Geometry: see drawing. Coordinates: mm, zero at the bounding-box minimum. A direction names the side the tool comes from. Give positions to 0.01 mm unless a question says otherwise; leave off trailing zeros. Loops run counter-clockwise (first coordinate to the right, second up) from the corner with the lowest first, then second, coordinate; pieces in that order, holes last. Notation, with made-up numbers: M -36,67 L -7,67 A24 ccw -7,90 Z; hole C -38,47.25 d6. An arc over 180 degrees is marked long. Put each result on its own line as item: value.
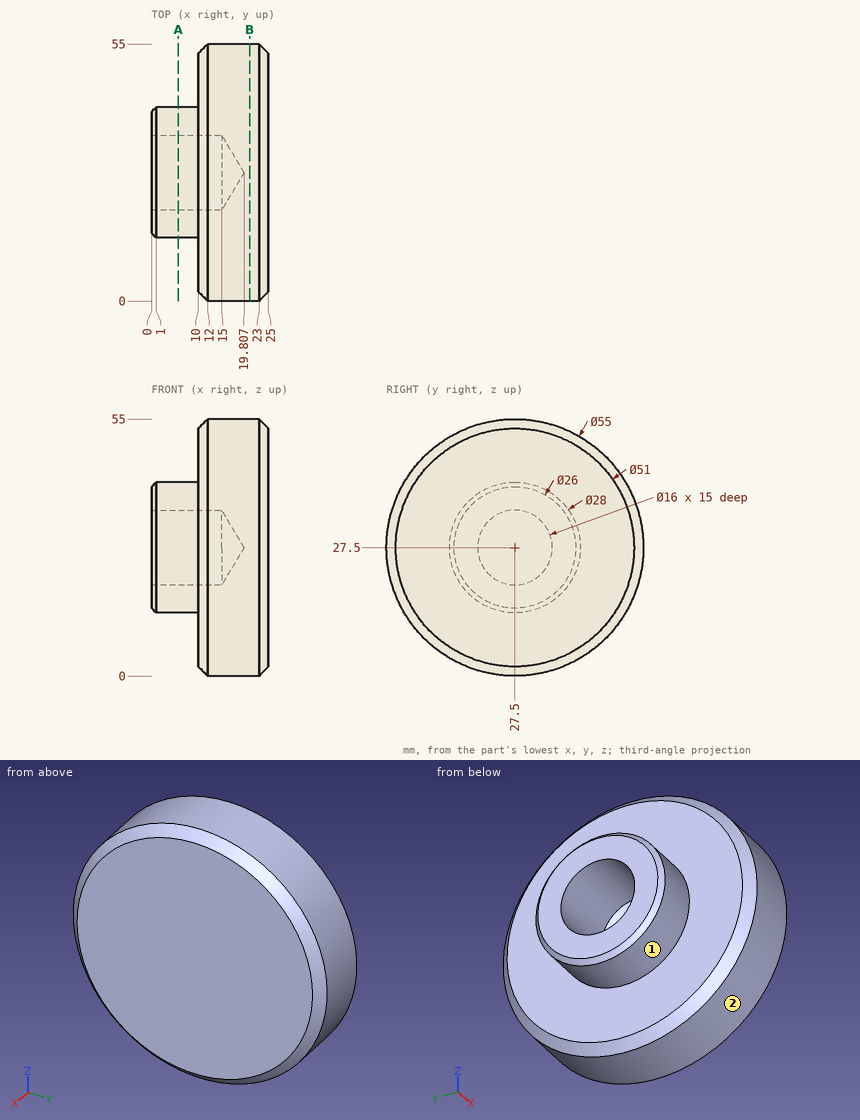
Item 1: Pin query (flat end, axial travel): pin 1 Ø6 at (x, z) = (8.5, 18.5) entering from +Y; pin 2 Ø10 at (x, y) = (18, 13.5) entering from -Z; pin 3 Ø3 at (x, z) = (13.5, 15.5) entering from -Y. Return the tip coordinate at first contact, or that it passes through.
Output values:
pin 1: y = 53.11
pin 2: z = 1.51
pin 3: y = 2.08
Item 2: Line query: probe 1 along Y at (x, z) = (6, 27.5); probe 2 along X at (y, z) = (15.5, 36.5); probe 3 along Z at (x, y) = (5, 28). Output: solid intervals per line, ascending. Write a range as [from, to].
Output values:
probe 1: [13.5, 19.5], [35.5, 41.5]
probe 2: [10, 25]
probe 3: [13.51, 19.52], [35.48, 41.49]
Item 3: Set-up query: the marked faces 1 and 2. Return all of +Z, -Z, +X, -X, +Y, -Y with unobstructed straight access to the full face (end or side cutting, diameter ignored); none if empty.
Output values:
face 1: -X
face 2: +X, -X
Item 4: Section A-A on x = 5.75. Output: boundary loops of the cut face in (y, z).
Output values:
outline: C 27.5,27.5 d28; hole C 27.5,27.5 d16
Item 5: Section B-B on x = 21. Output: boundary loops of the cut face in (y, z), then the cut area to 3 significant figures.
Output values:
outline: C 27.5,27.5 d55
area: 2,380 mm²
